Model file for the job. Use its own axes, mm. Face numbers are marked on the shaded views. A direction names the side the tool comes from. Give positions to 0.01 mm unless a question says otherwise; leave off trailing zeros. Write each loop counter-clockwise with the first axis right and the second up, starting at its lowest first coordinate (ties: lowest second). Pieces come first, ordered by that corner, then holes.
```python
from build123d import *

# Parameters (mm, degrees)
F0_W     = 220
F0_H     = 105
F1_DEPTH = 140
F2_W     = 200
F2_H     = 120
F3_DEPTH = 95
F5_DEPTH = 220.001


with BuildPart() as f1:
    # F0 (on Front) → F1 (new body)
    with BuildSketch(Plane.XZ):
        with Locations((110, 52.5)):
            Rectangle(F0_W, F0_H)
    extrude(amount=-F1_DEPTH)

    # F2 (on face) → F3 (cut)
    with BuildSketch(Plane.XY.offset(105)):
        with Locations((110, 70)):
            Rectangle(F2_W, F2_H)
    extrude(amount=-F3_DEPTH, mode=Mode.SUBTRACT)

    # F4 (on face) → F5 (cut, through all)
    with BuildSketch(Plane.YZ.offset(220)):
        with BuildLine():
            Line((95.4, 76), (44.6, 76))
            ThreePointArc((44.6, 76), (33.6, 65), (44.6, 54))
            Line((44.6, 54), (95.4, 54))
            ThreePointArc((95.4, 54), (106.4, 65), (95.4, 76))
        make_face()
    extrude(amount=-F5_DEPTH, mode=Mode.SUBTRACT)


solid = f1.part
```
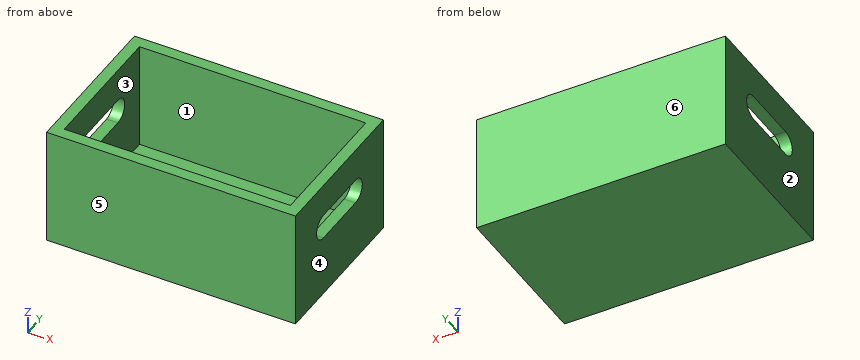
1. Which spindle directions (+Z, -Z, +X, -X, +Y, -Y) get a long thin tool onto all of the face, cutting with end or side? Do the marked faces 1 and 2. Say none if no direction does.
Calculated:
face 1: +Z
face 2: +Z, -Z, -X, +Y, -Y
2. Pin check, flat tip, straight feed: P1, Ø8, axis at x = 51.5, y = 49.5, coming from the +Z side. Stop position of the tip, or through.
Calculated:
P1: stops at z = 10
3. Slice it at D-D, the plane z = 40.5. Write the cut outline in (x, y).
Calculated:
outline: (0, 0) - (220, 0) - (220, 140) - (0, 140) - close; hole (10, 10) - (210, 10) - (210, 130) - (10, 130) - close
4. Slice it at B-B, the plane y = 49.5. Write the cut outline in (x, z).
Calculated:
outline: (0, 0) - (220, 0) - (220, 54) - (210, 54) - (210, 10) - (10, 10) - (10, 54) - (0, 54) - close; (0, 76) - (10, 76) - (10, 105) - (0, 105) - close; (210, 76) - (220, 76) - (220, 105) - (210, 105) - close
5. Slice it at C-C, the plane x = 75.5. Write the cut outline in (y, z), and give its area (3 significant figures).
Calculated:
outline: (0, 0) - (140, 0) - (140, 105) - (130, 105) - (130, 10) - (10, 10) - (10, 105) - (0, 105) - close
area: 3,300 mm2
6. Slice it at A-A, the plane z = 65. Write the cut outline in (x, y).
Calculated:
outline: (0, 0) - (220, 0) - (220, 33.6) - (210, 33.6) - (210, 10) - (10, 10) - (10, 33.6) - (0, 33.6) - close; (0, 106.4) - (10, 106.4) - (10, 130) - (210, 130) - (210, 106.4) - (220, 106.4) - (220, 140) - (0, 140) - close
7. Probe probe 1 along X at (y, z) = (22.5, 88); probe 2 along Y at (x, z) = (55.5, 68); probe 3 along Z at (x, y) = (121, 23). List the from-to ranges inside material, lowest first.
Calculated:
probe 1: x = 0 to 10, 210 to 220
probe 2: y = 0 to 10, 130 to 140
probe 3: z = 0 to 10
8. Pull direction Y, two halves, no side cores. Call the marked faces 3, 4, 5 and 6: +Y half, -Y half, draft (parallel to the pull), parting line (faces both ways), or undercut.
Calculated:
face 3: undercut
face 4: draft
face 5: -Y half
face 6: +Y half
